For this review, take the finished solid that the model builds, in its own axes (mm). Face numbers are marked on the shaded views. Round coordinates to 2 decimals unless told otherwise and drop trailing zeros. Loops run counter-clockwise (first coordinate to the right, second up) from the corner with the lowest first, then second, coordinate; pieces in that order, holes last.
1) Take a section at A-A (x = 3). State the section outline as (y, z) points, then the cut area to 3 significant figures.
2) Take a section at C-C (x = -36). State the section outline as (y, z) points.
3) Mouldability with a two-part tool opening along Z and no side actions: class the marked faces 1 and 2 as pulls with the +Z half, pulls with the -Z half, needs draft (parallel to the pull), parting line crosses it, or undercut.
4) Take a section at B-B (z = -4). State the section outline as (x, y) points, then the cut area to 3 significant figures.
5) Insertion check: pin 1 (4 mm diameter, centred on y = 2, z = 46.5, fed in from +X); pin 2 (1.5 mm diameter, centred on y = 8, z = -97.5, fed in from +X); pin 3 (5.5 mm diameter, centred on y = 2, z = 9.5, fed in from +X). Each pin has a flat end and moves straight along its axis. Give the tip position at first contact, or say it passes through.
6) Wall thickness on L1, parallel to Y at x = -22, z = -97; L2, parallel to Z at x = -5, y = 2; L3, parallel to Y at x = -21.5, z = -6: over which ranges is each line inside the solid? List them lowest first.
Autodesk Inventor part; units mm, degrees
ref_plane "Work Plane2" through (-55, 0, 0) normal (0, 0, 1) x (1, 0, 0)
ref_plane "YZ Plane" through (0, 0, 0) normal (1, 0, 0) x (0, 1, 0)
ref_plane "XZ Plane" through (0, 0, 0) normal (0, 1, 0) x (-1, 0, 0)
sketch "Sketch1" plane through (0, 0, 0) normal (0, 1, 0) x (-1, 0, 0)
  line L0 (11, 55) -> (-11, 55)
  line L1 (-11, 55) -> (-11, -55)
  line L2 (-11, -55) -> (11, -55)
  line L3 (11, -55) -> (11, 55)
  line L4 (11, 55) -> (-11, -55) construction
  line L5 (-11, 55) -> (11, -55) construction
  line L6 (55, 100) -> (-55, 100)
  line L7 (-55, 100) -> (-55, -100)
  line L8 (-55, -100) -> (55, -100)
  line L9 (55, -100) -> (55, 100)
  line L10 (55, 100) -> (-55, -100) construction
  line L11 (-55, 100) -> (55, -100) construction
  line L12 (55, 100) -> (7.4, 100)
  line L13 (7.4, 100) -> (7.4, 46.4)
  line L14 (7.4, 46.4) -> (55, 46.4)
  line L15 (55, 46.4) -> (55, 100)
  line L16 (55, 0) -> (11, 0)
  circle A0 centre (33, 0) radius 4
  line L17 (-11, -55) -> (-11, -100)
  circle A1 centre (0, -75) radius 5
  point P0 (0, 0)
  dimension "d0" = 22
  dimension "d1" = 110
  dimension "d2" = 200
  dimension "d3" = 110
  dimension "d6" = 53.6
  dimension "d7" = 47.6
  dimension "d12" = 8
  dimension "d17" = 10
  dimension "d20" = 20
extrude "Extrusion1" add sketch "Sketch1" along normal blind 5 contours L0 L13 L6 L9 L14 L3 | L0 L1 L17 L8 L7 L6 L13 | L14 L9 L16 A0 L3 | L16 A0 L9 L8 L17 L2 L3 | A0 L16 | L16 A0 | A1
sketch "Sketch3" plane through (0, 5, 0) normal (0, 1, 0) x (1, 0, 0)
  line L0 (11, 55) -> (11, -55)
  line L1 (11, -55) -> (11, -100)
  line L2 (-55, -100) -> (55, -100)
  line L3 (-11, 55) -> (11, 55)
  line L4 (11, 55) -> (11, 100)
  line L5 (55, 100) -> (-55, 100)
  line L6 (55, -100) -> (55, 100)
  point P0 (0, 0)
extrude "Extrusion3" cut sketch "Sketch3" against normal through all
sketch "Sketch4" plane through (0, 5, 0) normal (0, 1, 0) x (1, 0, 0)
  line L0 (-11, -55) -> (-11, 55)
  line L1 (-11, -55) -> (-21, -55)
  line L2 (-21, -55) -> (-21, -35)
  line L3 (-21, -35) -> (-11, -35)
  point P0 (0, 0)
  dimension "d21" = 10
  dimension "d22" = 20
extrude "Extrusion6" cut sketch "Sketch4" against normal through all
mirror "Mirror1" about plane through (0, 0, 0) normal (0, 0, 1) of "Extrusion6"
sketch "Sketch5" plane through (-55, 0, 100) normal (0, 0, 1) x (1, 0, 0)
  circle A0 centre (33, 10) radius 2.5
  circle A1 centre (33, 10) radius 5
  line L0 (66, 0) -> (66, 5)
  line L1 (0, 5) -> (66, 5)
  line L2 (0, 0) -> (0, 5)
  line L3 (0, 0) -> (66, 0)
  line L4 (0, 5) -> (66, 5)
  line L5 (38, 10) -> (38, 5)
  line L6 (66, 5) -> (0, 5)
  line L7 (33, 0) -> (33, 5)
  line L8 (28, 10) -> (28, 5)
  point P0 (55, 0)
  point P1 (38, 5)
  point P2 (33, 5)
  point P3 (28, 5)
  dimension "d25" = 5
  dimension "d26" = 10
extrude "Extrusion7" add sketch "Sketch5" against normal blind 5 contours A1 | L5 L1 A1 | A1 L1 L8
ref_plane "Work Plane2" through (-55, 0, 0) normal (0, 0, 1) x (1, 0, 0)
mirror "Mirror4" about plane through (-55, 0, 0) normal (0, 0, 1) of "Extrusion7"
properties part number "FP V2 Mounting Claw"
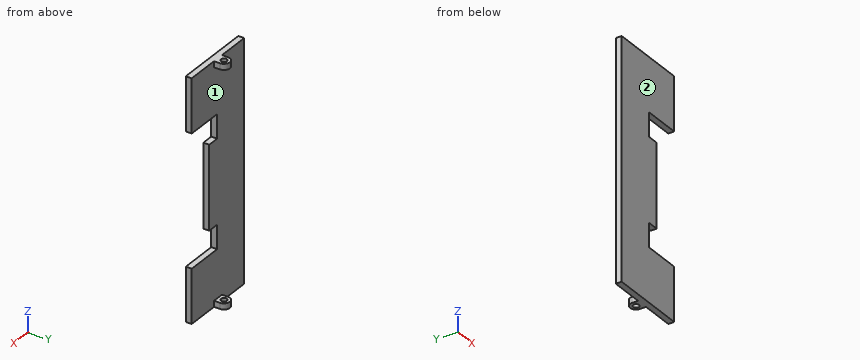
Response:
1. outline: (0, -100) - (5, -100) - (5, -55) - (0, -55) - close; (0, 55) - (5, 55) - (5, 100) - (0, 100) - close
1. area: 450 mm2
2. outline: (0, -100) - (5, -100) - (5, 100) - (0, 100) - close
3. face 1: undercut
3. face 2: needs draft
4. outline: (-55, 0) - (-11, 0) - (-11, 5) - (-55, 5) - close
4. area: 220 mm2
5. pin 1: stops at x = -21
5. pin 2: stops at x = -17
5. pin 3: stops at x = -11
6. L1: y = 0 to 7.5, 12.5 to 15
6. L2: z = -100 to -55, 55 to 100
6. L3: y = 0 to 5
